Geometry: final body of the model. Coordinates: model frame, mm. A direction names the side the tool comes from. Give positions to 0.01 mm unless a question says otherwise; leave off trailing zeros. Write each loop counter-clockwise with the first axis right and the second up, starting at its lowest first coordinate (ties: lowest second). Pieces come first, ordered by that corner, then holes. Notation, with made-up numbers: (69.5, 58) -> (105.5, 58) arc R18 cw to (105.5, 90) -> close; hole circle Ø3 at (4.5, 79.5). An arc over 180 degrees is marked (long way). Use CSV: the item, a comma, the result in double quotes. Start each with the question number.
1) Material intervals for line 1 (Z direction, x = -11.5, y = 3); line 2 (X direction, y = 0.65, z = 6.1); line 3 (X direction, y = 2.75, z = 0), sorted ascending. Write a range as [from, to].
2) Set-up query: faces 1 (the face through (0, 1, -10.263)), 2 (the face through (-2.74, 5.3, 1.95)), 3 (the face through (11, 1, -5.4)). Return all of +Z, -Z, +X, -X, +Y, -Y with unobstructed straight access to the full face (end or side cutting, diameter ignored); none if empty.
3) Contact query for flat-ended pins moving along their axis: P1, Ø2.5, axis at x = 4.52, z = -6.1, coming from the +Y side; P2, Ø1.5, axis at y = 8, z = -5.5, coming from the -X side; P3, Ø1, axis at y = 4.5, z = 0.5, coming from the -X side; P4, Ø2.5, axis at x = 4.52, z = 6.1, coming from the -Y side. Output: stop coordinate, or through.
4) Section C-C (y = 8.25). Output: boundary loops of the cut face in (x, z), plus the area to 3 significant figures.
5) Draft query along X for faces 4 (the face through (6.024, 1, 0)), 5 (the face through (0, 0, 0)), 6 (the face through (-23.049, 1, 0)). Return one class per face: pulls with the +X half, pulls with the -X half, needs draft (parallel to the pull), parting line crosses it, or undercut.
6) Section A-A (z = 0). Output: boundary loops of the cut face in (x, y), plus the area to 3 significant figures.
7) Section B-B (x = 8.5). Output: boundary loops of the cut face in (y, z), plus the area to 3 significant figures.
```python
from build123d import *

# Parameters (mm, degrees)
CROQUIS1_W              = 46.097746062
CROQUIS1_H              = 20.525775368
CROQUIS1_R              = 1.05
SALIENTE_EXTRUIR1_DEPTH = 1.5
CROQUIS4_W              = 11
CROQUIS4_H              = 10.8
CORTAR_EXTRUIR1_DEPTH   = 1.5
REDONDEO1_R             = 0.55
CROQUIS7_R              = 9
SALIENTE_EXTRUIR3_DEPTH = 7.7
CROQUIS8_R              = 8.2
CORTAR_EXTRUIR3_DEPTH   = 27.855491275
REDONDEO2_R             = 0.5
REDONDEO3_R             = 0.5


with BuildPart() as part:
    # Croquis1 → Saliente-Extruir1 (new body)
    with BuildSketch(Plane(origin=(0, 0, 0), x_dir=(1, 0, 0), z_dir=(0, 1, 0))):
        Rectangle(CROQUIS1_W, CROQUIS1_H)
        with Locations(Location((4.524436516, 6.1, 0), (0, 0, 270))):
            Circle(CROQUIS1_R, mode=Mode.SUBTRACT)
        with Locations(Location((18.524436516, 6.1, 0), (0, 0, 270))):
            Circle(CROQUIS1_R, mode=Mode.SUBTRACT)
        with Locations(Location((18.524436516, -6.1, 0), (0, 0, 90))):
            Circle(CROQUIS1_R, mode=Mode.SUBTRACT)
        with Locations(Location((4.524436516, -6.1, 0), (0, 0, 90))):
            Circle(CROQUIS1_R, mode=Mode.SUBTRACT)
    extrude(amount=SALIENTE_EXTRUIR1_DEPTH)

    # Croquis4 → Cortar-Extruir1 (cut)
    with BuildSketch(Plane(origin=(0, 1.5, 0), x_dir=(1, 0, 0), z_dir=(0, 1, 0))):
        with Locations((11.524436516, 0)):
            Rectangle(CROQUIS4_W, CROQUIS4_H)
    extrude(amount=-CORTAR_EXTRUIR1_DEPTH, mode=Mode.SUBTRACT)

    # Redondeo1
    redondeo1_edges = [part.edges().sort_by_distance(p)[0] for p in [
        (6.024436516, 0.75, -5.4),
        (17.024436516, 0.75, -5.4),
        (17.024436516, 0.75, 5.4),
        (6.024436516, 0.75, 5.4),
    ]]
    fillet(redondeo1_edges, radius=REDONDEO1_R)

    # Croquis7 → Saliente-Extruir3 (add)
    with BuildSketch(Plane(origin=(0, 1.5, 0), x_dir=(1, 0, 0), z_dir=(0, 1, 0))):
        with Locations(Location((-11.524436516, 0, 0), (0, 0, 90))):
            Circle(CROQUIS7_R)
    extrude(amount=SALIENTE_EXTRUIR3_DEPTH)

    # Croquis8 → Cortar-Extruir3 (cut, through all)
    with BuildSketch(Plane(origin=(0, 9.2, 0), x_dir=(1, 0, 0), z_dir=(0, 1, 0))):
        with Locations(Location((-11.524436516, 0, 0), (0, 0, 270))):
            Circle(CROQUIS8_R)
    extrude(amount=-CORTAR_EXTRUIR3_DEPTH, mode=Mode.SUBTRACT)

    # Redondeo2
    redondeo2_edges = [part.edges().sort_by_distance(p)[0] for p in [
        (17.024436516, 0, 0),
        (11.524436516, 0, 5.4),
        (6.024436516, 0, 0),
        (11.524436516, 0, -5.4),
        (16.863345245, 0, 5.23890873),
        (6.185527786, 0, 5.23890873),
        (16.863345245, 0, -5.23890873),
        (6.185527786, 0, -5.23890873),
    ]]
    fillet(redondeo2_edges, radius=REDONDEO2_R)

    # Redondeo3
    redondeo3_edges = [part.edges().sort_by_distance(p)[0] for p in [
        (-11.524436516, 0, -8.2),
    ]]
    fillet(redondeo3_edges, radius=REDONDEO3_R)


solid = part.part
```
Answers follow:
1,line 1,"z = [-9, -8.2], [8.2, 9]"
1,line 2,"x = [-23.05, -17], [-6.04, 3.47], [5.57, 17.47], [19.57, 23.05]"
1,line 3,"x = [-20.52, -19.72], [-3.32, -2.52]"
2,face 1,"-Z, +X, -X, +Y, -Y"
2,face 2,"+Y"
2,face 3,"+Y, -Y"
3,P1,"stops at y = 1.5"
3,P2,"stops at x = -19.17"
3,P3,"stops at x = -20.52"
3,P4,"stops at y = 0"
4,outline,"circle Ø18 at (-11.52, 0); hole circle Ø16.4 at (-11.52, 0)"
4,area,"43.2 mm^2"
5,face 4,"undercut"
5,face 5,"needs draft"
5,face 6,"pulls with the -X half"
6,outline,"(-23.05, 0) -> (-20.22, 0) arc R0.5 ccw to (-19.72, 0.5) -> (-19.72, 9.2) -> (-20.52, 9.2) -> (-20.52, 1.5) -> (-23.05, 1.5) -> close; (-3.32, 0.5) arc R0.5 ccw to (-2.82, 0) -> (5.52, 0) arc R0.5 ccw to (6.02, 0.5) -> (6.02, 1.5) -> (-2.52, 1.5) -> (-2.52, 9.2) -> (-3.32, 9.2) -> close; (17.02, 0.5) arc R0.5 ccw to (17.52, 0) -> (23.05, 0) -> (23.05, 1.5) -> (17.02, 1.5) -> close"
6,area,"40.2 mm^2"
7,outline,"(0, -10.26) -> (1.5, -10.26) -> (1.5, -5.4) -> (0.5, -5.4) arc R0.5 ccw to (0, -5.9) -> close; (0, 5.9) arc R0.5 ccw to (0.5, 5.4) -> (1.5, 5.4) -> (1.5, 10.26) -> (0, 10.26) -> close"
7,area,"14.5 mm^2"
